For this review, take the finished solid that the model builds, in its own axes (mm). A direction names the side the tool comes from. Coordinates: 2 decimals unless noted, no trailing zeros. Write each loop counter-clockwise with the first axis right and the second up, starting at its lowest first coordinate (ties: lowest second). Pieces come first, ordered by that corner, then holes. Notation, with made-up numbers: M -20.75,81 L 34.25,81 A26 ccw 34.25,96 Z; hole C 11,-23 d1. An arc over 180 degrees is marked long. Return JSON: item names as keys, results as strings.
Autodesk Inventor part; units mm, degrees
ref_plane "Work Plane2" through (0, 0, 5) normal (0, 0, 1) x (1, 0, 0)
ref_plane "Work Plane8" through (0, 0, 0) normal (0.8660254, 0.5, 0) x (0, 0, 1)
ref_plane "Work Plane9" through (0, 0, 0) normal (1, 0, 0) x (0, 1, 0)
sketch "Sketch1" plane through (0, 0, 0) normal (0, 0, 1) x (1, 0, 0)
  circle A0 centre (0, 0) radius 7.688
  dimension "d0" = 15.376
extrude "Extrusion1" add sketch "Sketch1" along normal blind 10
ref_plane "Work Plane2" through (0, 0, 5) normal (0, 0, 1) x (1, 0, 0)
sketch "Sketch2" plane through (0, 0, 0) normal (0, 0, -1) x (-1, 0, 0)
  circle A0 centre (0, 0) radius 7.688
  circle A1 centre (0, 0) radius 6
  dimension "d3" = 12
surface extrude "Pitch Diameter" sketch "Sketch2" against normal through all shown no curves A1
ref_plane "Work Plane8" through (0, 0, 0) normal (0.8660254, 0.5, 0) x (0, 0, 1)
ref_plane "Work Plane9" through (0, 0, 0) normal (1, 0, 0) x (0, 1, 0)
spur gear teeth "Spur Gear" teeth 6 pitch diameter 12 tip diameter 15.376 root diameter 7 face width 10 start plane through (0, 0, 0) normal (0, 0, -1) x (-1, 0, 0)
equation "\"d0\" = da_da"
equation "\"d1\" = da_b"
equation "\"d3\" = da_d"
properties part number "Spur Gear1" material "Steel"
1. Wall thickness on L1, parallel to X at y = 4, z = 2; L2, parallel to X at y = 3.75, z = 5.75; L3, parallel to Y at x = -5, z = 2.25: over which ranges is each line inside the solid? List them lowest first. Write a range as from..to.
Checks:
{"L1": "-6.57..-3.87, -1.48..1.48, 3.87..6.57", "L2": "-6.71..-3.41, -1.45..1.45, 3.41..6.71", "L3": "-4.45..-1.1, 1.1..4.45"}
2. Draft analysis for pull direction X (two halves, no side actions). For faces 5 (the face through (3.99, -4.06, 4.93)), 6 (the face through (6.65, 3.86, 4.93)), 7 (the face through (-6.665, 3.832, 4.93)), state which applies: +X half, -X half, draft (parallel to the pull), parting line (faces both ways), or undercut.
Checks:
{"face 5": "undercut", "face 6": "+X half", "face 7": "-X half"}
3. We need section C-C (x = 4.5). State the section outline as (y, z) points, plus the area to 3 significant figures.
Checks:
{"outline": "M -4.28,0 L -0.84,0 L -0.84,10 L -4.28,10 Z; M 0.84,0 L 4.28,0 L 4.28,10 L 0.84,10 Z", "area": "68.7 mm2"}
4. Clearance check with flat-ended pins moving along their axes: pin 1 Ø1 at (y, z) = (-5, 2.5) entering from +X; pin 2 Ø6 at (x, z) = (-5.5, 2.5) entering from +Y; pin 3 Ø1.5 at (x, z) = (-5.5, 3.5) entering from -Y. State where each tip first meets the part, or that it passes through.
Checks:
{"pin 1": "x = 6.23", "pin 2": "y = 4.68", "pin 3": "y = -4.68"}
5. For faces 1 (the face through (-3.93, -4.03, 4.93)), 2 (the face through (-3.99, 4.06, 4.93)), 3 (the face through (5.512, 1.426, 4.93)), 4 (the face through (-1.52, -5.49, 4.93)), list the 3-axis set-ups (+Z, -Z, +X, -X, +Y, -Y) from which the entire face can be reached by the end or side of a thin tool; tool diameter is ignored.
Checks:
{"face 1": "+Z, -Z, -Y", "face 2": "+Z, -Z, +Y", "face 3": "+Z, -Z, +X", "face 4": "+Z, -Z"}
6. We need section B-B (x = -5). State the section outline as (y, z) points.
Checks:
{"outline": "M -4.45,0 L -1.1,0 L -1.1,10 L -4.45,10 Z; M 1.1,0 L 4.45,0 L 4.45,10 L 1.1,10 Z"}
7. We need section A-A (z = 7.75). State the section outline as (x, y) points.
Checks:
{"outline": "M -7.1,-2.94 A7.69 ccw -6.1,-4.68 A7.04 ccw -2.13,-2.78 A3.5 ccw -1.34,-3.23 A7.04 ccw -1,-7.62 A7.69 ccw 1,-7.62 A7.04 ccw 1.34,-3.23 A3.5 ccw 2.13,-2.78 A7.04 ccw 6.1,-4.68 A7.69 ccw 7.1,-2.94 A7.04 ccw 3.47,-0.46 A3.5 ccw 3.47,0.46 A7.04 ccw 7.1,2.94 A7.69 ccw 6.1,4.68 A7.04 ccw 2.13,2.78 A3.5 ccw 1.34,3.23 A7.04 ccw 1,7.62 A7.69 ccw -1,7.62 A7.04 ccw -1.34,3.23 A3.5 ccw -2.13,2.78 A7.04 ccw -6.1,4.68 A7.69 ccw -7.1,2.94 A7.04 ccw -3.47,0.46 A3.5 ccw -3.47,-0.46 A7.04 ccw Z"}
8. We need section D-D (y = 6.5). State the section outline as (x, z) points, plus the area to 3 significant figures.
Checks:
{"outline": "M -1.36,0 L 1.36,0 L 1.36,10 L -1.36,10 Z", "area": "27.3 mm2"}
